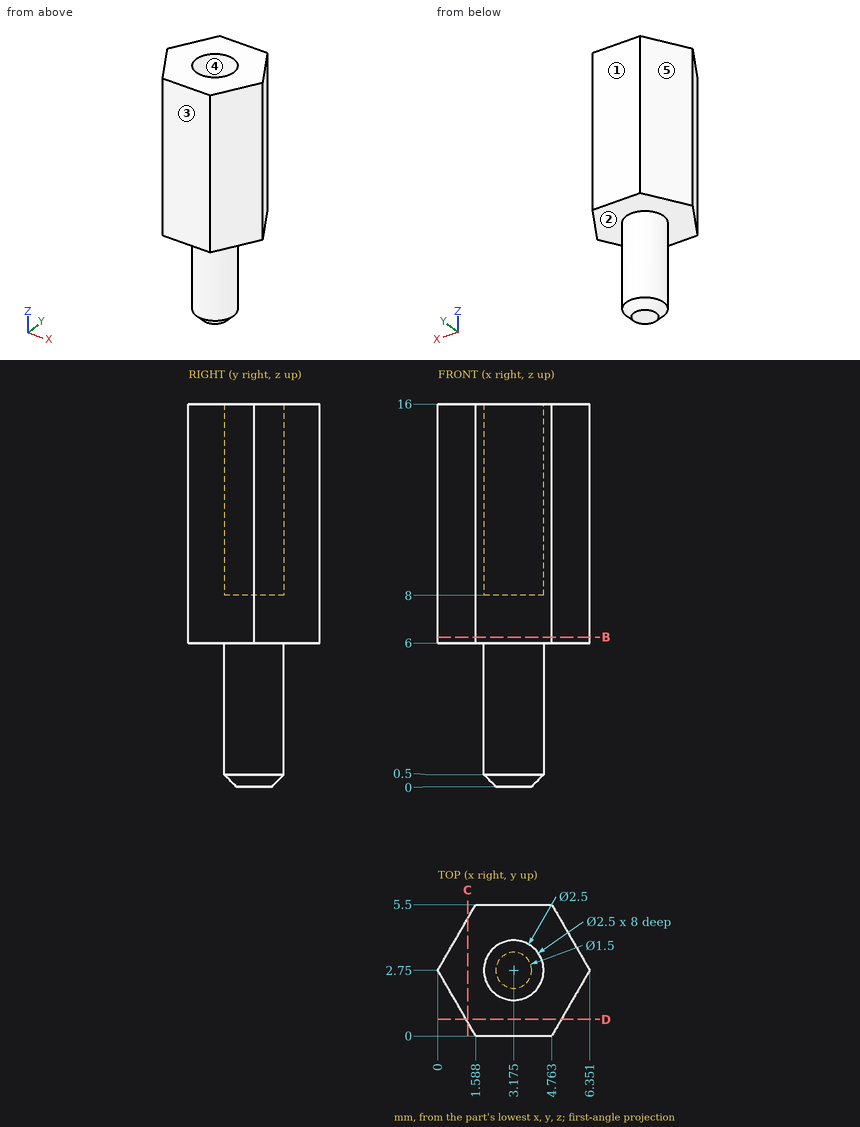
For this review, use the dimensioned drawing (mm, ordinates from the lowest corner) and the shaded views. A direction names the side the tool comes from. Give positions to 0.01 mm unless a question says otherwise; leave off trailing zeros. Loops run counter-clockwise (first coordinate to the right, second up) from the corner with the lowest first, then second, coordinate; pieces in that order, holes last.
Item 1: Take a section at B-B, the plane z = 6.25. State the section outline as (x, y) points.
Item 2: For line 1 along Z through (x, y) = (4.25, 1.5); line 2 along Y through (x, z) = (2.5, 8.5); line 3 along Y through (x, z) = (3, 12.25), list the stretches that pass through material, from the lowest coordinate up.
Item 3: Take a section at C-C, the plane x = 1.25. State the section outline as (y, z) points (1 decimal).
Item 4: Take a section at D-D, the plane y = 0.7. State the section outline as (x, z) points.
Item 5: Tool access review of the marked faces 1 and 2: name each direction out of +Z, -Z, +X, -X, +Y, -Y from which nothing blocks a thin tool from reaching the whole face with its end or side.
Item 6: Insertion check: pin 1 (2 mm diameter, centred on x = 3.18, y = 2.75, fed in from +Z). The pin has a flat end and moves straight along its axis. Give the tip position at first contact, or say it passes through.
Item 7: Draft analysis for pull direction X (two halves, no side actions). For the marked faces 3, 4 and 5, state which applies: +X half, -X half, draft (parallel to the pull), parting line (faces both ways), or undercut.
Calculated:
1. outline: (0, 2.75) - (1.59, 0) - (4.76, 0) - (6.35, 2.75) - (4.76, 5.5) - (1.59, 5.5) - close
2. line 1: z = 6 to 16
2. line 2: y = 0 to 1.7, 3.8 to 5.5
2. line 3: y = 0 to 1.51, 3.99 to 5.5
3. outline: (0.6, 6) - (4.9, 6) - (4.9, 16) - (0.6, 16) - close
4. outline: (1.18, 6) - (5.17, 6) - (5.17, 16) - (1.18, 16) - close
5. face 1: +Z, -Z, +X, -X, +Y
5. face 2: -Z
6. pin 1: stops at z = 8
7. face 3: draft
7. face 4: undercut
7. face 5: -X half
